The model under review builds one solid part; all positions refer to its coordinate system, in mm. Coordinates: 2 decimals unless noted, no trailing zeros. Order: outer loops, then holes, each group sorted by start corner. A loop starts at its lowest first (then second) coordinate and runs counter-clockwise, first axis right, second up. Notation, with made-up numbers: (10.5, 6) - (64.5, 6) arc R23 cw to (64.5, 30) - close; hole circle Ø6 at (34.5, 15). An arc over 180 degrees is marked (long way). Answer in a Markdown table with one row per item.
Autodesk Inventor part; units mm, degrees
ref_plane "YZ Plane" through (0, 0, 0) normal (1, 0, 0) x (0, 1, 0)
ref_plane "XZ Plane" through (0, 0, 0) normal (0, 1, 0) x (-1, 0, 0)
ref_plane "XY Plane" through (0, 0, 0) normal (0, 0, 1) x (1, 0, 0)
sketch "Sketch1" plane through (0, 0, 0) normal (0, 0, 1) x (1, 0, 0)
  line L0 (0, 0) -> (-165, 0)
  line L1 (-165, 0) -> (-165, 90)
  line L2 (-165, 90) -> (0, 90)
  line L3 (0, 90) -> (0, 0)
  line L4 (-165, 90) -> (-44, 90)
  line L5 (-44, 90) -> (-44, 40)
  line L6 (-44, 40) -> (-165, 40)
  line L7 (-165, 40) -> (-165, 90)
  dimension "d0" = 165
  dimension "d1" = 90
  dimension "d2" = 121
  dimension "d3" = 50
extrude "Extrusion1" add sketch "Sketch1" along normal blind 7 contours L0 L1 L6 L5 L2 L3
sketch "Sketch2" plane through (0, 0, 7) normal (0, 0, 1) x (1, 0, 0)
  circle A0 centre (-10, 76.0401) radius 1.5
  line L0 (0, 90) -> (-44, 90)
  line L1 (-22, 90) -> (-22, 0)
  circle A1 centre (-34, 76.0401) radius 1.5
  circle A2 centre (-10, 16.0401) radius 1.5
  circle A3 centre (-34, 16.0401) radius 1.5
  circle A4 centre (-145, 21) radius 1.5
  line L2 (-165, 40) -> (-165, 0)
  line L3 (-44, 40) -> (-165, 40)
  line L4 (-165, 0) -> (0, 0)
  dimension "d6" = 3
  dimension "d7" = 24
  dimension "d8" = 3
  dimension "d9" = 60
  dimension "d10" = 3
  dimension "d11" = 20
  dimension "d15" = 21
extrude "Extrusion2" cut sketch "Sketch2" against normal blind 10
sketch "Sketch3" plane through (0, 0, 7) normal (0, 0, 1) x (1, 0, 0)
  circle A0 centre (-10, 16.0401) radius 1.5
  circle A1 centre (-10, 16.0401) radius 3
  line L0 (0, 90) -> (-44, 90)
  line L1 (-22, 90) -> (-22, 0)
  line L2 (-165, 0) -> (0, 0)
  line L3 (-22, 90) -> (68, 90) construction
  circle A2 centre (-10, 76.0401) radius 1.5
  circle A3 centre (-10, 76.0401) radius 3
  circle A4 centre (-34, 16.0401) radius 3
  circle A5 centre (-34, 76.0401) radius 3
  circle A6 centre (-145, 21) radius 1.5
  circle A7 centre (-145, 21) radius 3
  dimension "d16" = 6
  dimension "d17" = 90
  dimension "d18" = 6
  dimension "d19" = 6
extrude "Extrusion3" cut sketch "Sketch3" against normal blind 4
properties part number "alt platform"
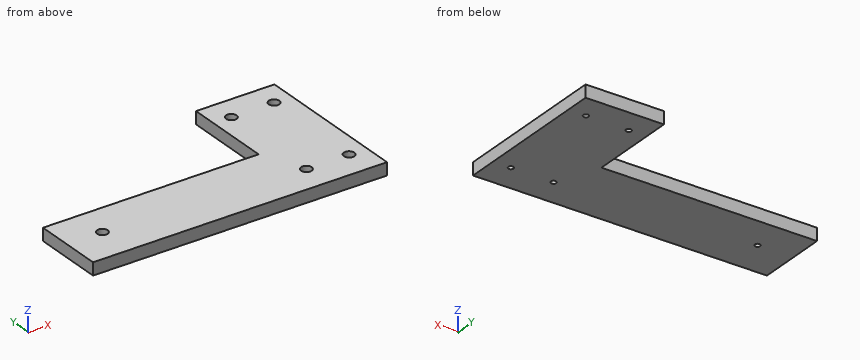
Item 1: We need section C-C, the plane y = 81. Write out the cut boundary in (x, z), then the cut area to 3 significant figures.
Check values:
| item | result |
|---|---|
| outline | (-44, 0) - (0, 0) - (0, 7) - (-44, 7) - close |
| area | 308 mm^2 |
Item 2: To check wall thickness, follow line 1 (Y direction, x = -10, z = 4.5); line 2 (Y direction, x = -145, z = 5.2); line 3 (X direction, y = 51.5, z = 6). State the ranges of each line that lie inside material, in increasing order. Write a range as from..to.
Check values:
| item | result |
|---|---|
| line 1 | 0..13.04, 19.04..73.04, 79.04..90 |
| line 2 | 0..18, 24..40 |
| line 3 | -44..0 |
Item 3: We need section A-A, the plane z = 1.75. Write out the cut boundary in (x, y).
Check values:
| item | result |
|---|---|
| outline | (-165, 0) - (0, 0) - (0, 90) - (-44, 90) - (-44, 40) - (-165, 40) - close; hole circle Ø3 at (-145, 21); hole circle Ø3 at (-34, 16.04); hole circle Ø3 at (-34, 76.04); hole circle Ø3 at (-10, 16.04); hole circle Ø3 at (-10, 76.04) |
Item 4: We need section B-B, the plane x = -93.5. Write out the cut boundary in (y, z), then the cut area to 3 significant figures.
Check values:
| item | result |
|---|---|
| outline | (0, 0) - (40, 0) - (40, 7) - (0, 7) - close |
| area | 280 mm^2 |
Item 5: Clearance check with flat-ended pins moving along their axes: pin 1 Ø3 at (x, y) = (-9, 76) entering from +Z; pin 2 Ø2 at (y, z) = (45.5, 2.5) entering from -X; pin 3 Ø1.5 at (x, z) = (-79, 2) entering from +Y. State where each tip first meets the part, or that it passes through.
Check values:
| item | result |
|---|---|
| pin 1 | z = 3 |
| pin 2 | x = -44 |
| pin 3 | y = 40 |
